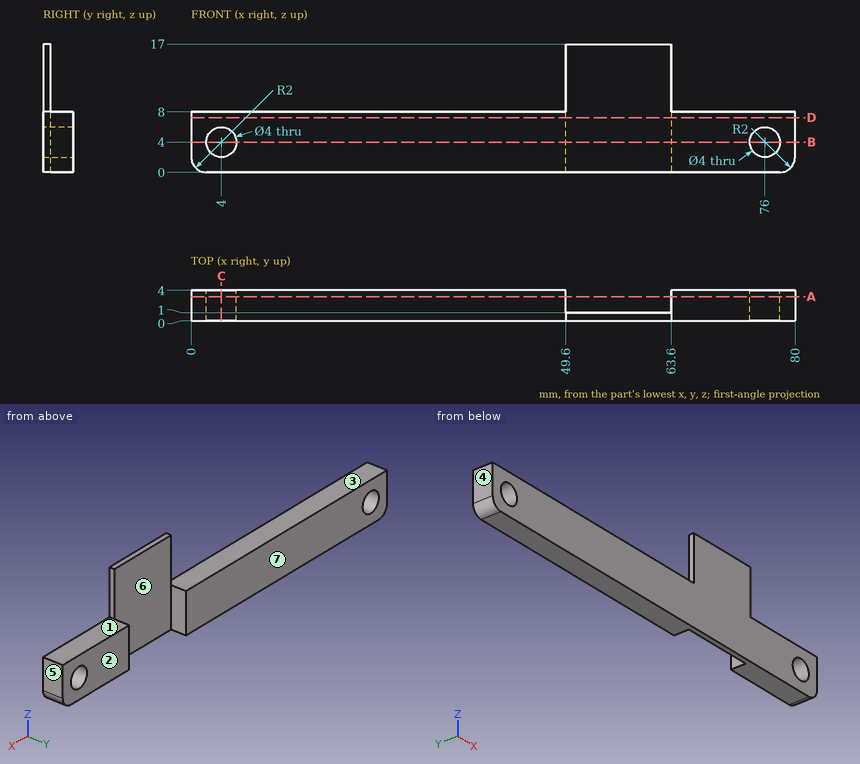
Design review of the part shown in the three views and the two pictorial views. Dimensions are in mm from the part's minimum x, y and z. A direction names the side the tool comes from. Coordinates: 2 decimals unless noted, no trailing zeros. Write each loop counter-clockwise with the first axis right and the second up, starting at its lowest first coordinate (ties: lowest second). Pieces come first, ordered by that corner, then holes.
1) We need section B-B on z = 4. State the section outline as (x, y) points.
2) Machinability: for the marked faces 1, 2 and 3, which of the approach directions +Z, -Z, +X, -X, +Y, -Y give a long, thin tool a straight path to every point of the face, cutting with its end or side? Answer none if there is none.
3) We need section A-A on y = 3.15. State the section outline as (x, z) points, then the cut area to 3 significant figures.
4) We need section C-C on x = 4. State the section outline as (y, z) points, then the cut area to 3 significant figures.
5) Clearance check with flat-ended pins moving along their axes: pin 1 Ø1.2 at (x, y) = (23, 3) entering from +Z; pin 2 Ø4 at (x, z) = (57.5, 6) entering from +Y; pin 3 Ø0.8 at (y, z) = (0.5, 11) entering from -X; pin 4 Ø3 at (x, z) = (76, 4) entering from -Y. State where each tip first meets the part, or that it passes through.
6) We need section D-D on z = 7.25. State the section outline as (x, y) points, then the cut area to 3 significant figures.
7) The part is to be moulded in two halves that separate along X. For the marked faces 4, 5, 6 and 7, say which applies: pulls with the +X half, pulls with the -X half, needs draft (parallel to the pull), parting line crosses it, or undercut.
8) To check wall thickness, follow probe 1 along X at (y, z) = (2.2, 4); probe 2 along X at (y, z) = (3.8, 6.5); probe 3 along Z at (x, y) = (76, 1.9). State the ranges of each line that lie inside material, in increasing order.
Answer list:
1. outline: (0, 0) - (2, 0) - (2, 4) - (0, 4) - close; (6, 0) - (74, 0) - (74, 4) - (63.6, 4) - (63.6, 1) - (49.6, 1) - (49.6, 4) - (6, 4) - close; (78, 0) - (80, 0) - (80, 4) - (78, 4) - close
2. face 1: +Z, +X, +Y, -Y
2. face 2: +Z, -Z, +X, -X, +Y
2. face 3: +Z, -X, +Y, -Y
3. outline: (0, 2) arc R2 ccw to (2, 0) - (49.6, 0) - (49.6, 8) - (0, 8) - close; (63.6, 0) - (78, 0) arc R2 ccw to (80, 2) - (80, 8) - (63.6, 8) - close; hole circle Ø4 at (4, 4); hole circle Ø4 at (76, 4)
3. area: 501 mm2
4. outline: (0, 0) - (4, 0) - (4, 2) - (0, 2) - close; (0, 6) - (4, 6) - (4, 8) - (0, 8) - close
4. area: 16.0 mm2
5. pin 1: stops at z = 8
5. pin 2: stops at y = 1
5. pin 3: stops at x = 49.6
5. pin 4: passes through
6. outline: (0, 0) - (80, 0) - (80, 4) - (63.6, 4) - (63.6, 1) - (49.6, 1) - (49.6, 4) - (0, 4) - close
6. area: 278 mm2
7. face 4: pulls with the -X half
7. face 5: pulls with the +X half
7. face 6: undercut
7. face 7: needs draft
8. probe 1: x = 0 to 2, 6 to 49.6, 63.6 to 74, 78 to 80
8. probe 2: x = 0 to 49.6, 63.6 to 80
8. probe 3: z = 0 to 2, 6 to 8
